from build123d import *

# Parameters (mm, degrees)
F0_W      = 210
F0_H      = 60
F1_DEPTH  = 2
F2_R      = 15
F3_DEPTH  = 2
F4_R      = 2
F5_DEPTH  = 2.5
F6_R      = 1.3
F7_DEPTH  = 2
F8_R      = 1.3
F9_DEPTH  = 2
F10_R     = 1.3
F11_DEPTH = 2
F12_R     = 1.3
F13_DEPTH = 2
F14_R     = 1.3
F15_DEPTH = 2
F16_R     = 1.3
F17_DEPTH = 2


with BuildPart() as f1:
    # F0 (on Top) → F1 (new body)
    with BuildSketch(Plane.XY):
        Rectangle(F0_W, F0_H)
    extrude(amount=F1_DEPTH)

    # F2 (on face) → F3 (cut)
    with BuildSketch(Plane.XY.offset(2)):
        with Locations((-88, 0)):
            Circle(F2_R)
        with Locations((-56, 0)):
            Circle(F2_R)
        with Locations((-16, 0)):
            Circle(F2_R)
        with Locations((16, 0)):
            Circle(F2_R)
        with Locations((56, 0)):
            Circle(F2_R)
        with Locations((88, 0)):
            Circle(F2_R)
    extrude(amount=-F3_DEPTH, mode=Mode.SUBTRACT)

    # F4 (on face) → F5 (join)
    with BuildSketch(Plane.XY.offset(2)):
        with Locations((-102, -27)):
            Circle(F4_R)
        with Locations((-102, 27)):
            Circle(F4_R)
        with Locations((102, -27)):
            Circle(F4_R)
        with Locations((102, 27)):
            Circle(F4_R)
        with Locations((0, 27)):
            Circle(F4_R)
        with Locations((0, -27)):
            Circle(F4_R)
    extrude(amount=F5_DEPTH)

    # F6 (on face) → F7 (cut)
    with BuildSketch(Plane.XY.offset(4.5)):
        with Locations((0, -27)):
            Circle(F6_R)
    extrude(amount=-F7_DEPTH, mode=Mode.SUBTRACT)

    # F8 (on face) → F9 (cut)
    with BuildSketch(Plane.XY.offset(4.5)):
        with Locations((-102, -27)):
            Circle(F8_R)
    extrude(amount=-F9_DEPTH, mode=Mode.SUBTRACT)

    # F10 (on face) → F11 (cut)
    with BuildSketch(Plane.XY.offset(4.5)):
        with Locations((-102, 27)):
            Circle(F10_R)
    extrude(amount=-F11_DEPTH, mode=Mode.SUBTRACT)

    # F12 (on face) → F13 (cut)
    with BuildSketch(Plane.XY.offset(4.5)):
        with Locations((0, 27)):
            Circle(F12_R)
    extrude(amount=-F13_DEPTH, mode=Mode.SUBTRACT)

    # F14 (on face) → F15 (cut)
    with BuildSketch(Plane.XY.offset(4.5)):
        with Locations((102, 27)):
            Circle(F14_R)
    extrude(amount=-F15_DEPTH, mode=Mode.SUBTRACT)

    # F16 (on face) → F17 (cut)
    with BuildSketch(Plane.XY.offset(4.5)):
        with Locations((102, -27)):
            Circle(F16_R)
    extrude(amount=-F17_DEPTH, mode=Mode.SUBTRACT)


solid = f1.part
Source: CAD feature listing. Evaluate the final solid. Frame: model axes, mm. A direction names the side the tool comes from. Round coordinates to 2 decimals unless told otherwise and drop trailing zeros. Write each loop counter-clockwise with the first axis right and the second up, starting at its lowest first coordinate (ties: lowest second). Pieces come first, ordered by that corner, then holes. Notation, with made-up numbers: M 52.25,31 L 73.25,31 A22 cw 73.25,57 Z; hole C 14,39.25 d8. An arc over 180 degrees is marked long. One line per item, written item: value. Start each with the question number.
Item 1: Ray query, L1, parallel to Y at x = 102, z = 3.4; L2, parallel to Y at x = 1.5, z = 3.95; L3, parallel to Z at x = -93.5, y = -15.5. Return the intervals inside material, ascending. Write a range as from..to.
Item 2: Section query D-D (x = -68.5). Return the cut outline in (y, z).
Item 3: Section query B-B (x = 68). Return the cut outline in (y, z).
Item 4: Mould query, pull axis Y, two halves, no side actions, for faces 1 (the cylindrical face through (-100.153, -27.766, 3.232)), 2 (the flat face through (-1, 7, 0)). Classes: pulls with the +Y half, pulls with the -Y half, needs draft (parallel to the pull), parting line crosses it, or undercut.
Item 5: Pin query (flat end, axial travel): pin 1 (18 mm diameter, centred on x = 88, y = 0, fed in from +Z); pin 2 (1.3 mm diameter, centred on x = 0, y = -27.5, fed in from +Z); pin 3 (1.5 mm diameter, centred on x = 21.5, y = 19, fed in from +Z). Return the tip coordinate at first contact, or that it passes through.
Item 6: Set-up query: faces 3 (the cylindrical face through (102.307, 4.506, 1.014)), 4 (the cylindrical face through (103.847, 26.234, 3.232)). Return all of +Z, -Z, +X, -X, +Y, -Y with unobstructed straight access to the full face (end or side cutting, diameter ignored); none if empty.
Item 7: Section query A-A (z = 3.7). State how many separate pieces and enclosed holes the cut face has, plus the area to 3 significant figures.
Item 8: Section query C-C (y = -4). Return the cut outline in (x, z), plus the area to 3 significant figures.
Result set:
1. L1: y = -29..-28.3, -25.7..-25, 25..25.7, 28.3..29
1. L2: y = -28.32..-25.68, 25.68..28.32
1. L3: z = 0..2
2. outline: M -30,0 L -8.29,0 L -8.29,2 L -30,2 Z; M 8.29,0 L 30,0 L 30,2 L 8.29,2 Z
3. outline: M -30,0 L -9,0 L -9,2 L -30,2 Z; M 9,0 L 30,0 L 30,2 L 9,2 Z
4. face 1: undercut
4. face 2: needs draft
5. pin 1: passes through
5. pin 2: stops at z = 2.5
5. pin 3: stops at z = 2
6. face 3: +Z, -Z
6. face 4: +Z
7. separate pieces: 6
7. enclosed holes: 6
7. area: 43.5 mm²
8. outline: M -105,0 L -102.46,0 L -102.46,2 L -105,2 Z; M -73.54,0 L -70.46,0 L -70.46,2 L -73.54,2 Z; M -41.54,0 L -30.46,0 L -30.46,2 L -41.54,2 Z; M -1.54,0 L 1.54,0 L 1.54,2 L -1.54,2 Z; M 30.46,0 L 41.54,0 L 41.54,2 L 30.46,2 Z; M 70.46,0 L 73.54,0 L 73.54,2 L 70.46,2 Z; M 102.46,0 L 105,0 L 105,2 L 102.46,2 Z
8. area: 73.0 mm²
